Geometry check sheet. Reference: the model listing, model coordinates, mm. Round coordinates to 2 decimals unless told otherwise and drop trailing zeros. Write each loop counter-clockwise with the first axis right and the second up, starting at its lowest first coordinate (ties: lowest second). Pieces come first, ordered by that corner, then holes. Notation, with made-up numbers: (-15.75, 85) -> (-2.75, 85) arc R19 ccw to (-2.75, 98) -> close; hole circle Ø7 at (54.5, -18.75). An arc over 180 degrees is marked (long way). Use a Markdown table: item, result.
Autodesk Inventor part; units mm, degrees
ref_plane "YZ Plane" through (0, 0, 0) normal (1, 0, 0) x (0, 1, 0)
ref_plane "XZ Plane" through (0, 0, 0) normal (0, 1, 0) x (-1, 0, 0)
ref_plane "XY Plane" through (0, 0, 0) normal (0, 0, 1) x (1, 0, 0)
sketch "Sketch1" plane through (0, 0, 0) normal (0, 0, 1) x (1, 0, 0)
  circle A0 centre (0, 0) radius 15
  line L0 (-73.4722, 0) -> (96.5278, 0) construction
  line L1 (0, 0) -> (0, 31) construction
  circle A1 centre (0, 0) radius 1.5
  circle A2 centre (-6.9148, 6.9148) radius 1.7526
  line L2 (0, 0) -> (-14.5685, 14.5685) construction
  circle A3 centre (-6.9148, -6.9148) radius 1.7526
  circle A4 centre (6.9148, -6.9148) radius 1.7526
  circle A5 centre (6.9148, 6.9148) radius 1.7526
  point P0 (0, 0)
  dimension "d4" = 30
  dimension "d10" = 3
  dimension "d11" = 3.5052
  dimension "d12" = 45
  dimension "d13" = 6.9148
  dimension "d16" = 360
extrude "Extrusion1" add sketch "Sketch1" along normal blind 5 contours A0 | A1 | A2 | A3 | A4 | A5
extrude "Extrusion2" cut sketch "Sketch1" along normal through all contours A1 | A2 | A3 | A4 | A5
equation "\"BendRadius\" = Thickness"
equation "\"BendReliefWidth\" = Thickness"
equation "\"BendReliefDepth\" = 0.5 * Thickness"
equation "\"CornerReliefSize\" = 4 * Thickness"
equation "\"MinimumRemnant\" = 2 * Thickness"
equation "\"TransitionRadius\" = BendRadius"
equation "\"JacobiRadiusSize\" = Thickness"
equation "\"GapSize\" = Thickness"
properties part number "encoder_spacer"
(1) Section check D-D on z = 3.6. Record the cut outline in (x, y), plus the area to 3 significant figures.
A:
| item | result |
|---|---|
| outline | circle Ø30 at (0, 0); hole circle Ø3.51 at (-6.91, -6.91); hole circle Ø3.51 at (-6.91, 6.91); hole circle Ø3 at (0, 0); hole circle Ø3.51 at (6.91, -6.91); hole circle Ø3.51 at (6.91, 6.91) |
| area | 661 mm2 |
(2) Thickness scan on line 1 (X direction, y = 6, z = 3.35); line 2 (X direction, y = -7.25, z = 1.05). Record the ranges inside material, lowest first.
A:
| item | result |
|---|---|
| line 1 | x = -13.75 to -8.41, -5.42 to 5.42, 8.41 to 13.75 |
| line 2 | x = -13.13 to -8.64, -5.19 to 5.19, 8.64 to 13.13 |
(3) Section check A-A on x = 0. Record the cut outline in (y, z).
A:
| item | result |
|---|---|
| outline | (-15, 0) -> (-1.5, 0) -> (-1.5, 5) -> (-15, 5) -> close; (1.5, 0) -> (15, 0) -> (15, 5) -> (1.5, 5) -> close |
(4) Gauge pin test, flat ends, axial feed: pin 1 Ø2 at (x, y) = (6.91, -6.91) entering from -Z; pin 2 Ø3 at (x, z) = (-8, 2.5) entering from +Y; pin 3 Ø1.5 at (y, z) = (9.5, 1) entering from -X. Record the tip position at first contact, or that the pin passes through.
A:
| item | result |
|---|---|
| pin 1 | passes through |
| pin 2 | stops at y = 13.52 |
| pin 3 | stops at x = -12.18 |
(5) Section check C-C on y = -6. Record the cut outline in (x, z).
A:
| item | result |
|---|---|
| outline | (-13.75, 0) -> (-8.41, 0) -> (-8.41, 5) -> (-13.75, 5) -> close; (-5.42, 0) -> (5.42, 0) -> (5.42, 5) -> (-5.42, 5) -> close; (8.41, 0) -> (13.75, 0) -> (13.75, 5) -> (8.41, 5) -> close |
(6) Release check for a two-part mould opening along X. For faces 1 (the face through (-14.985, -0.66, 2.465)), 2 (the face through (6.535, 8.626, 2.465)), 3 (the face through (0, -3, 5)) record: +X half, -X half, draft (parallel to the pull), parting line (faces both ways), or undercut.
A:
| item | result |
|---|---|
| face 1 | parting line |
| face 2 | undercut |
| face 3 | draft |
